Can you work these out from the model? Positions are in its coordinate system, mm. Face numbers are marked on the shaded views. Coordinates: 2 decimals unless noted, no trailing zeros. Order: outer loops, then holes, each group sorted by start corner. A loop starts at its lowest first (then second) coordinate and runs counter-clockwise, first axis right, second up. Notation, with made-up numbers: M 88.5,2 L 95.5,2 A18 cw 95.5,34 Z; hole C 18.25,-3 d5. An arc over 180 degrees is marked long. Answer as CSV lines item,"result". Start each with the question number.
1. Will these pins go through, and if not, where does the flat tip stop? pin 1 (4 mm diameter, centred on x = -6.5, y = 20, fed in from -Z); pin 2 (8 mm diameter, centred on x = 12, y = 32, fed in from +Z); pin 3 (6 mm diameter, centred on x = -14, y = 41, fed in from +Z); pin 4 (3 mm diameter, centred on x = -0.5, y = 27.5, fed in from +Z).
2. If we section it at B-B (x = 0): List the corners of the cut face in (y, z) for me.
3. If we mould it in two halves opening along Z, with no side actions, what happens to the marked faces 1 and 2? For each: released by +Z, released by -Z, zero draft, split by the parting line, or undercut.
4. If we section it at C-C (y = 34.5): List the corners of the cut face in (x, z) for me, plus the area to 3 significant figures.
5. I need wall thicknesses on line 1 along X through (y, z) = (19.5, 0); line 2 along Y through (x, z) = (-8.5, -0.5); line 3 along X through (y, z) = (17, 11.5). Which ranges of each line are inside material? Lowest first, please. Write a range as from..to.
6. If we section it at A-A (z = 0): List the corners of the cut face in (x, y) for me, plus the area to 3 significant figures.
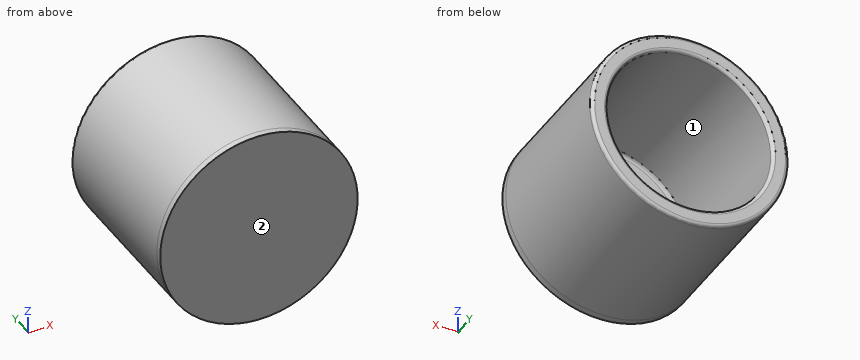
```python
from build123d import *

# Parameters (mm, degrees)
SKETCH1_R           = 30
SKETCH1_R_2         = 25
BOSS_EXTRUDE1_DEPTH = 50
BOSS_EXTRUDE2_START = 2
SKETCH2_R           = 30
BOSS_EXTRUDE2_DEPTH = 2
FILLET1_R           = 1


with BuildPart() as part:
    # Sketch1 → Boss-Extrude1 (new body)
    with BuildSketch(Plane(origin=(0, 0, 0), x_dir=(1, 0, 0), z_dir=(0, 1, 0))):
        with Locations(Location((0, 0, 0), (0, 0, 270))):
            Circle(SKETCH1_R)
        with Locations(Location((0, 0, 0), (0, 0, 270))):
            Circle(SKETCH1_R_2, mode=Mode.SUBTRACT)
    extrude(amount=BOSS_EXTRUDE1_DEPTH)

    # Sketch2 → Boss-Extrude2 (add)
    with BuildSketch(Plane.XZ.offset(BOSS_EXTRUDE2_START)):
        with Locations(Location((0, 0, 0), (0, 0, 270))):
            Circle(SKETCH2_R)
    extrude(amount=-BOSS_EXTRUDE2_DEPTH)

    # Fillet1
    fillet1_edges = [part.edges().sort_by_distance(p)[0] for p in [
        (0, 50, -30),
        (0, 0, -25),
        (0, 50, -25),
    ]]
    fillet(fillet1_edges, radius=FILLET1_R)


solid = part.part
```
Solved:
1,pin 1,"z = -29.66"
1,pin 2,"z = 28.91"
1,pin 3,"z = 27.91"
1,pin 4,"z = 30"
2,outline,"M -2,-30 L 49,-30 A1 ccw 50,-29 L 50,-26 A1 ccw 49,-25 L 1,-25 A1 cw 0,-24 L 0,24 A1 cw 1,25 L 49,25 A1 ccw 50,26 L 50,29 A1 ccw 49,30 L -2,30 Z"
3,face 1,"undercut"
3,face 2,"zero draft"
4,outline,"C 0,0 d60; hole C 0,0 d50"
4,area,"864 mm²"
5,line 1,"-30..-25, 25..30"
5,line 2,"-2..0"
5,line 3,"-27.71..-22.2, 22.2..27.71"
6,outline,"M -30,-2 L 30,-2 L 30,49 A1 ccw 29,50 L 26,50 A1 ccw 25,49 L 25,1 A1 cw 24,0 L -24,0 A1 cw -25,1 L -25,49 A1 ccw -26,50 L -29,50 A1 ccw -30,49 Z"
6,area,"620 mm²"
